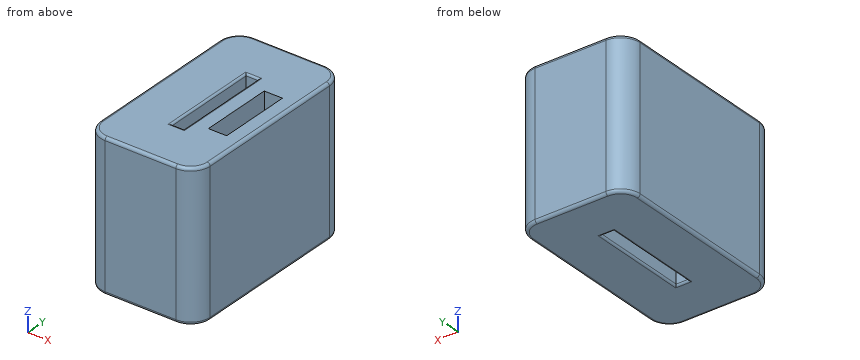
```python
from build123d import *

# Parameters (mm, degrees)
SKETCH1_W           = 28.6258
SKETCH1_H           = 50.8508
SKETCH1_W_2         = 3.2258
SKETCH1_H_2         = 25.4508
BOSS_EXTRUDE1_DEPTH = 19.05
FILLET1_R           = 5.08
FILLET3_R           = 0.762
FILLET4_R           = 0.508
SKETCH2_R           = 9.525
CUT_EXTRUDE1_DEPTH  = 3.175
CUT_EXTRUDE2_DEPTH  = 2.38125


with BuildPart() as part:
    # Sketch1 → Boss-Extrude1 (new, symmetric)
    with BuildSketch(Plane.XY):
        Rectangle(SKETCH1_W, SKETCH1_H)
        Rectangle(SKETCH1_W_2, SKETCH1_H_2, mode=Mode.SUBTRACT)
    extrude(amount=BOSS_EXTRUDE1_DEPTH, both=True)

    # Fillet1
    fillet1_edges = [part.edges().sort_by_distance(p)[0] for p in [
        (-14.3129, -25.4254, 0),
        (-14.3129, 25.4254, 0),
        (14.3129, 25.4254, 0),
        (14.3129, -25.4254, 0),
    ]]
    fillet(fillet1_edges, radius=FILLET1_R)

    # Fillet3
    fillet3_edges = [part.edges().sort_by_distance(p)[0] for p in [
        (0, -25.4254, -19.05),
        (0, -25.4254, 19.05),
        (-14.3129, 0, -19.05),
        (0, 25.4254, -19.05),
        (14.3129, 0, -19.05),
        (12.825002448, 23.937502448, -19.05),
        (-12.825002448, 23.937502448, -19.05),
        (12.825002448, -23.937502448, -19.05),
        (-12.825002448, -23.937502448, -19.05),
        (-14.3129, 0, 19.05),
        (14.3129, 0, 19.05),
        (0, 25.4254, 19.05),
        (12.825002448, 23.937502448, 19.05),
        (-12.825002448, 23.937502448, 19.05),
        (12.825002448, -23.937502448, 19.05),
        (-12.825002448, -23.937502448, 19.05),
    ]]
    fillet(fillet3_edges, radius=FILLET3_R)

    # Fillet4
    fillet4_edges = [part.edges().sort_by_distance(p)[0] for p in [
        (1.6129, 0, -19.05),
        (0, 12.7254, -19.05),
        (-1.6129, 0, -19.05),
        (0, -12.7254, -19.05),
        (1.6129, 0, 19.05),
        (0, 12.7254, 19.05),
        (-1.6129, 0, 19.05),
        (0, -12.7254, 19.05),
    ]]
    fillet(fillet4_edges, radius=FILLET4_R)

    # Sketch2 → Cut-Extrude1 (cut, symmetric)
    with BuildSketch(Plane(origin=(7.9629, 0, 0), x_dir=(0, 0, -1), z_dir=(1, 0, 0))):
        Circle(SKETCH2_R)
    extrude(amount=CUT_EXTRUDE1_DEPTH, both=True, mode=Mode.SUBTRACT)

    # Sketch2_3 → Cut-Extrude2 (cut, symmetric)
    with BuildSketch(Plane(origin=(7.9629, 0, 0), x_dir=(0, 0, -1), z_dir=(1, 0, 0))):
        with BuildLine():
            ThreePointArc((0, -9.525), (-9.525, 0), (0, 9.525))
            Line((0, 9.525), (-19.05, 9.525))
            Line((-19.05, 9.525), (-19.05, -9.525))
            Line((-19.05, -9.525), (0, -9.525))
        make_face()
    extrude(amount=CUT_EXTRUDE2_DEPTH, both=True, mode=Mode.SUBTRACT)


solid = part.part
```
Part model, mm, in its own coordinate system. Coordinates: 2 decimals unless noted, no trailing zeros. Order: outer loops, then holes, each group sorted by start corner. A loop starts at its lowest first (then second) coordinate and runs counter-clockwise, first axis right, second up. Notation, with made-up numbers: (77, 72) -> (89, 72) arc R27 cw to (89, 97) -> close; hole circle Ø1 at (34, -20). An arc over 180 degrees is marked (long way). Put each result on its own line as item: value. Start each with the question number.
(1) Band-saw the part on A-A (y = -11). Give the cut face in (x, z), then the cut area to 3 significant figures.
(2) Probe line 1 along X through (y, z) = (3, 16.5); line 2 along X through (y, z) = (5, -8); line 3 along Y through (x, z) = (8, 0) (3 decimals). List the from-to ranges inside material, lowest first. Write a range as [from, to].
(3) Band-saw the part on C-C (z = -11). Give the cut face in (x, y).
(4) Band-saw the part on D-D (y = 0). Give the cut face in (x, z) (3 decimals), then the cut area to 3 significant figures.
(5) Band-saw the part on B-B (z = 14). Give the cut face in (x, y) (3 decimals).
Determined:
1. outline: (-14.31, -18.29) arc R0.76 ccw to (-13.55, -19.05) -> (-2.12, -19.05) arc R0.51 ccw to (-1.61, -18.54) -> (-1.61, 18.54) arc R0.51 ccw to (-2.12, 19.05) -> (-13.55, 19.05) arc R0.76 ccw to (-14.31, 18.29) -> close; (1.61, -18.54) arc R0.51 ccw to (2.12, -19.05) -> (13.55, -19.05) arc R0.76 ccw to (14.31, -18.29) -> (14.31, 18.29) arc R0.76 ccw to (13.55, 19.05) -> (2.12, 19.05) arc R0.51 ccw to (1.61, 18.54) -> close
1. area: 967 mm²
2. line 1: x = [-14.31, -1.61], [1.61, 5.58], [10.34, 14.31]
2. line 2: x = [-14.31, -1.61], [1.61, 4.79], [11.14, 14.31]
2. line 3: y = [-25.425, -9.525], [9.525, 25.425]
3. outline: (-14.31, -20.35) arc R5.08 ccw to (-9.23, -25.43) -> (9.23, -25.43) arc R5.08 ccw to (14.31, -20.35) -> (14.31, 20.35) arc R5.08 ccw to (9.23, 25.43) -> (-9.23, 25.43) arc R5.08 ccw to (-14.31, 20.35) -> close; hole (-1.61, -12.73) -> (1.61, -12.73) -> (1.61, 12.73) -> (-1.61, 12.73) -> close
4. outline: (-14.313, -18.288) arc R0.762 ccw to (-13.551, -19.05) -> (-2.121, -19.05) arc R0.508 ccw to (-1.613, -18.542) -> (-1.613, 18.542) arc R0.508 ccw to (-2.121, 19.05) -> (-13.551, 19.05) arc R0.762 ccw to (-14.313, 18.288) -> close; (1.613, -18.542) arc R0.508 ccw to (2.121, -19.05) -> (13.551, -19.05) arc R0.762 ccw to (14.313, -18.288) -> (14.313, 18.288) arc R0.762 ccw to (13.551, 19.05) -> (10.344, 19.05) -> (10.344, 9.525) -> (11.138, 9.525) -> (11.138, -9.525) -> (4.788, -9.525) -> (4.788, 9.525) -> (5.582, 9.525) -> (5.582, 19.05) -> (2.121, 19.05) arc R0.508 ccw to (1.613, 18.542) -> close
4. area: 801 mm²
5. outline: (-14.313, -20.345) arc R5.08 ccw to (-9.233, -25.425) -> (9.233, -25.425) arc R5.08 ccw to (14.313, -20.345) -> (14.313, 20.345) arc R5.08 ccw to (9.233, 25.425) -> (-9.233, 25.425) arc R5.08 ccw to (-14.313, 20.345) -> close; hole (-1.613, -12.725) -> (1.613, -12.725) -> (1.613, 12.725) -> (-1.613, 12.725) -> close; hole (5.582, -9.525) -> (10.344, -9.525) -> (10.344, 9.525) -> (5.582, 9.525) -> close
